```python
from build123d import *

# Parameters (mm, degrees)
SKETCH1_R               = 20
BOSS_EXTRUDE1_DEPTH     = 3
SKETCH2_R               = 7.5
BOSS_EXTRUDE2_DEPTH     = 10
SKETCH6_W               = 6
SKETCH6_H               = 16
BOSS_EXTRUDE3_DEPTH     = 10
SKETCH3_R               = 4.5
CUT_EXTRUDE1_DEPTH      = 32.128764833
SKETCH4_R               = 1.75
CUT_EXTRUDE2_DEPTH      = 31
CUT_EXTRUDE3_DEPTH      = 32.128764833
CUT_EXTRUDE3_DEPTH_BACK = 32.128764833
SKETCH5_R               = 1.75


with BuildPart() as part:
    # Sketch1 → Boss-Extrude1 (new body)
    with BuildSketch(Plane.XY):
        Circle(SKETCH1_R)
    extrude(amount=BOSS_EXTRUDE1_DEPTH)

    # Sketch2 → Boss-Extrude2 (add)
    with BuildSketch(Plane.XY.offset(3)):
        Circle(SKETCH2_R)
    extrude(amount=BOSS_EXTRUDE2_DEPTH)

    # Sketch6 → Boss-Extrude3 (add)
    with BuildSketch(Plane.XY.offset(3)):
        Rectangle(SKETCH6_W, SKETCH6_H)
    extrude(amount=BOSS_EXTRUDE3_DEPTH)

    # Sketch3 → Cut-Extrude1 (cut, through all)
    with BuildSketch(Plane.XY.offset(13)):
        Circle(SKETCH3_R)
    extrude(amount=-CUT_EXTRUDE1_DEPTH, mode=Mode.SUBTRACT)

    # Sketch4 → Cut-Extrude2 (cut, through all)
    with BuildSketch(Plane.XY.offset(3)):
        with Locations((0, 15)):
            Circle(SKETCH4_R)
        with Locations((10.606601718, 10.606601718)):
            Circle(SKETCH4_R)
        with Locations((15, 0)):
            Circle(SKETCH4_R)
        with Locations((10.606601718, -10.606601718)):
            Circle(SKETCH4_R)
        with Locations((0, -15)):
            Circle(SKETCH4_R)
        with Locations((-10.606601718, -10.606601718)):
            Circle(SKETCH4_R)
        with Locations((-15, 0)):
            Circle(SKETCH4_R)
        with Locations((-10.606601718, 10.606601718)):
            Circle(SKETCH4_R)
    extrude(amount=-CUT_EXTRUDE2_DEPTH, mode=Mode.SUBTRACT)

    # Sketch5 → Cut-Extrude3 (cut, two sides: drawn at the far end of the back side and taken through both)
    with BuildSketch(Plane(origin=(0, 0, 0), x_dir=(1, 0, 0), z_dir=(0, 1, 0)).offset(-CUT_EXTRUDE3_DEPTH_BACK)):
        with Locations(Location((0, -8, 0), (0, 0, 270))):
            Circle(SKETCH5_R)
    extrude(amount=CUT_EXTRUDE3_DEPTH + CUT_EXTRUDE3_DEPTH_BACK, mode=Mode.SUBTRACT)


solid = part.part
```
CAD build for the part. Positions are in the model's coordinates, mm. A direction names the side the tool comes from. Coordinates: 2 decimals unless noted, no trailing zeros. Write each loop counter-clockwise with the first axis right and the second up, starting at its lowest first coordinate (ties: lowest second). Pieces come first, ordered by that corner, then holes. Notation, with made-up numbers: (82, 45.25) -> (104, 45.25) arc R21 cw to (104, 50.25) -> close; hole circle Ø4 at (55.25, 64.25). An arc over 180 degrees is marked (long way). Use CSV: the item, a comma, the result in double quotes. Start each with the question number.
Item 1: Tool access for faces 5 (the flat face through (2, 8, 8)), 6 (the flat face through (3, 7.4, 7.9)), 7 (the cylindrical face through (-7.5, 0.1, 7.9)), 8 (the flat face through (-3, -7.4, 7.9)): list every direction of +Z, -Z, +X, -X, +Y, -Y with a clear straight run to the whole face (end or side of a thin tool).
Item 2: Band-saw the part on A-A, the plane z = 8. Write the cut outline in (x, y), plus the area to 3 significant figures.
Item 3: Drop flat-ended pins along their axis: P1, Ø11.5, axis at x = 0, y = 0, coming from the -Z side; P2, Ø3, axis at x = -1, z = 6, coming from the +Y side; P3, Ø0.9, axis at y = 7, z = 9.5, coming from the -X side; P4, Ø5.5, axis at x = 10.61, y = -10.61, coming from the +Z side. Give the stop position or say it passes through.
Item 4: Band-saw the part on B-B, the plane x = 0. Write the cut outline in (y, z).
Item 5: Band-saw the part on D-D, the plane y = 15. Write the cut outline in (x, z).
Item 6: Wall check: probe 1 along Y at (x, z) = (0, 2.15); probe 2 along Y at (x, z) = (9.5, 2.5); probe 3 along X at (y, z) = (12, 2.25). Give the ranges that are in metal, low to high.
Item 7: Two-plate mould, pull along Z, no slides. Class faces 1 (the cylindrical face through (0.526, 6.046, 9.669)), 2 (the flat face through (0, -9, 3)), 3 (the cylindrical face through (0.08, -6.1, 6.25)), 4 (the flat face through (-3, 7.4, 7.9)): +Z half, -Z half, draft (parallel to the pull), parting line (faces both ways), or undercut.
Item 8: Band-saw the part on C-C, the plane y = 0. Write the cut outline in (x, z).
Response values:
1,face 5,"+Z, +X, -X, +Y"
1,face 6,"+Z, +X, +Y"
1,face 7,"+Z, -X"
1,face 8,"+Z, -X, -Y"
2,outline,"(-3, -8) -> (-1.75, -8) -> (-1.75, -4.15) arc R4.5 cw to (-1.75, 4.15) -> (-1.75, 8) -> (-3, 8) -> (-3, 6.87) arc R7.5 ccw to (-3, -6.87) -> close; (1.75, -8) -> (3, -8) -> (3, -6.87) arc R7.5 ccw to (3, 6.87) -> (3, 8) -> (1.75, 8) -> (1.75, 4.15) arc R4.5 cw to (1.75, -4.15) -> close"
2,area,"96.2 mm2"
3,P1,"stops at z = 0"
3,P2,"stops at y = 8"
3,P3,"stops at x = -3.65"
3,P4,"stops at z = 3"
4,outline,"(-20, 0) -> (-16.75, 0) -> (-16.75, 3) -> (-20, 3) -> close; (-13.25, 0) -> (-4.5, 0) -> (-4.5, 6.25) -> (-8, 6.25) -> (-8, 3) -> (-13.25, 3) -> close; (-8, 9.75) -> (-4.5, 9.75) -> (-4.5, 13) -> (-8, 13) -> close; (4.5, 0) -> (13.25, 0) -> (13.25, 3) -> (8, 3) -> (8, 6.25) -> (4.5, 6.25) -> close; (4.5, 9.75) -> (8, 9.75) -> (8, 13) -> (4.5, 13) -> close; (16.75, 0) -> (20, 0) -> (20, 3) -> (16.75, 3) -> close"
5,outline,"(-13.23, 0) -> (-1.75, 0) -> (-1.75, 3) -> (-13.23, 3) -> close; (1.75, 0) -> (13.23, 0) -> (13.23, 3) -> (1.75, 3) -> close"
6,probe 1,"y = -20 to -16.75, -13.25 to -4.5, 4.5 to 13.25, 16.75 to 20"
6,probe 2,"y = -17.6 to -11.96, -9.25 to 9.25, 11.96 to 17.6"
6,probe 3,"x = -16 to -11.67, -9.55 to 9.55, 11.67 to 16"
7,face 1,"undercut"
7,face 2,"+Z half"
7,face 3,"undercut"
7,face 4,"draft"
8,outline,"(-20, 0) -> (-16.75, 0) -> (-16.75, 3) -> (-20, 3) -> close; (-13.25, 0) -> (-4.5, 0) -> (-4.5, 13) -> (-7.5, 13) -> (-7.5, 3) -> (-13.25, 3) -> close; (4.5, 0) -> (13.25, 0) -> (13.25, 3) -> (7.5, 3) -> (7.5, 13) -> (4.5, 13) -> close; (16.75, 0) -> (20, 0) -> (20, 3) -> (16.75, 3) -> close"
